from build123d import *

# Parameters (mm, degrees)
F0_R     = 55
F1_DEPTH = 19
F2_W     = 5.214504
F2_H     = 5
F2_W_2   = 59
F2_H_2   = 33
F3_DEPTH = 17
F4_W     = 6
F4_H     = 11
F4_W_2   = 11
F4_H_2   = 16
F4_W_3   = 5
F4_H_3   = 10
F5_DEPTH = 19.001


with BuildPart() as f1:
    # F0 (on Top) → F1 (new body)
    with BuildSketch(Plane.XY):
        Circle(F0_R)
    extrude(amount=F1_DEPTH)

    # F2 (on face) → F3 (cut)
    with BuildSketch(Plane.XY.offset(19)):
        Polygon((52.392748, 2.5), (52.392748, 8), (14.392748, 8), (14.392748, -8), (52.392748, -8), (52.392748, -2.5), align=None)
        with Locations((55, 0)):
            Rectangle(F2_W, F2_H)
        with Locations((0, 26.5)):
            Rectangle(F2_W_2, F2_H_2)
        with Locations((0, -26.5)):
            Rectangle(F2_W_2, F2_H_2)
        Polygon((-14.392748, 8), (-52.392748, 8), (-52.392748, 2.5), (-52.392748, -2.5), (-52.392748, -8), (-14.392748, -8), align=None)
        with Locations((-55, 0)):
            Rectangle(F2_W, F2_H)
    extrude(amount=-F3_DEPTH, mode=Mode.SUBTRACT)

    # F4 (on face) → F5 (cut, through all)
    with BuildSketch(Plane.XY.offset(19)):
        with Locations((-34.5, 15.5)):
            Rectangle(F4_W, F4_H)
        with Locations((34.5, 15.5)):
            Rectangle(F4_W, F4_H)
        with Locations((-5.5, 50.5)):
            Rectangle(F4_W, F4_H)
        with Locations((5.5, 50.5)):
            Rectangle(F4_W, F4_H)
        with Locations((-19.892748, 0)):
            Rectangle(F4_W_2, F4_H_2)
        with Locations((19.892748, 0)):
            Rectangle(F4_W_2, F4_H_2)
        with Locations((27, 26.5)):
            Rectangle(F4_W_3, F4_H_3)
        with Locations((-27, 26.5)):
            Rectangle(F4_W_3, F4_H_3)
        with Locations((27, -26.5)):
            Rectangle(F4_W_3, F4_H_3)
        with Locations((-27, -26.5)):
            Rectangle(F4_W_3, F4_H_3)
    extrude(amount=-F5_DEPTH, mode=Mode.SUBTRACT)


solid = f1.part
The model under review builds one solid part; all positions refer to its coordinate system, in mm. A direction names the side the tool comes from. Give positions to 0.01 mm unless a question says otherwise; leave off trailing zeros. Write each loop counter-clockwise with the first axis right and the second up, starting at its lowest first coordinate (ties: lowest second). Pieces come first, ordered by that corner, then holes.
1. Add section C-C, the plane y = 0. Write out the cut boundary in (x, z), plus the area to 3 significant figures.
2. For P1, Ø6.5, axis at x = -6, z = 12, coming from the +Y side; P2, Ø5, axis at y = -13, z = 15, coming from the +X side; P3, Ø1.6, axis at y = -6.5, z = 8, coming from the +X side; P4, Ø8.5, axis at x = -3.5, z = 12.5, coming from the -Y side, all flat-tipped, find the tip position at first contact; note any pin that passes through.
3. Add section A-A, the plane y = -24. Write out the cut boundary in (x, z).
4. Tool access review of faces 4 (the flat face through (52.393, -5, 11)), 5 (the flat face through (-54, 2.5, 11)), 6 (the flat face through (-31.5, 15, 10)): name each direction out of +Z, -Z, +X, -X, +Y, -Y from which nothing blocks a thin tool from reaching the whole face with its end or side.
5. Add section D-D, the plane z = 6. Count the separate pieces of the cut face and the enclosed holes in it, plus the area to 3 significant figures.
6. Add section B-B, the plane x = 0. Write out the cut boundary in (y, z), plus the area to 3 significant figures.
7. Wall thickness on L1, parallel to Y at x = 0, z = 7; L2, parallel to Y at x = 18.5, z = 8; L3, parallel to Y at x = 32, z = 17.75: over which ranges is each line inside the solid? List them lowest first.
8. Draft analysis for pull direction Y (two halves, no side actions). For faces 1 (the flat face through (2.5, 50, 10)), 2 (the flat face through (-29.5, 26, 10)), 3 (the cylindrical face through (-2.3, -54.95, 9.37)), state which applies: +Y half, -Y half, draft (parallel to the pull), parting line (faces both ways), or undercut.
Worked answers:
1. outline: (-55, 0) - (-25.39, 0) - (-25.39, 2) - (-55, 2) - close; (-14.39, 0) - (14.39, 0) - (14.39, 19) - (-14.39, 19) - close; (25.39, 0) - (55, 0) - (55, 2) - (25.39, 2) - close
1. area: 665 mm2
2. P1: stops at y = 54.34
2. P2: stops at x = 53.99
2. P3: stops at x = 54.7
2. P4: stops at y = -55
3. outline: (-49.49, 0) - (-29.5, 0) - (-29.5, 19) - (-49.49, 19) - close; (-24.5, 0) - (24.5, 0) - (24.5, 2) - (-24.5, 2) - close; (29.5, 0) - (49.49, 0) - (49.49, 19) - (29.5, 19) - close
4. face 4: +Z
4. face 5: +Z, -X
4. face 6: +Z, -Z
5. separate pieces: 1
5. enclosed holes: 4
5. area: 4,120 mm2
6. outline: (-55, 0) - (55, 0) - (55, 19) - (43, 19) - (43, 2) - (10, 2) - (10, 19) - (-10, 19) - (-10, 2) - (-43, 2) - (-43, 19) - (-55, 19) - close
6. area: 968 mm2
7. L1: y = -55 to -43, -10 to 10, 43 to 55
7. L2: y = -51.8 to -43, -10 to -8, 8 to 10, 43 to 51.8
7. L3: y = -44.73 to -8, 8 to 10, 21 to 44.73
8. face 1: draft
8. face 2: undercut
8. face 3: parting line
